Can you work these out from the model? Positions are in its coordinate system, mm. Face numbers are marked on the shaded views. Give positions to 0.01 mm unless a question says otherwise; leave off trailing zeros. Loops run counter-clockwise (first coordinate to the right, second up) from the corner with the lowest first, then second, coordinate; pieces in that order, holes last. Notation, with made-up numbers: (59.5, 48.5) -> (71.5, 48.5) arc R20 cw to (71.5, 76.5) -> close; hole circle Ø5 at (-5, 63.5). An arc over 180 degrees is marked (long way). Return JSON: item names as keys, results as strings. Group by question number.
Q1. Suppose I cut it at B-B, the plane y = 35. Please give me the cut outline in (x, z), and give its area (3 significant figures).
Q2. Thinking about a two-plate mould opening in X: for the marked faces 1 and 2, which applies, pulls with the +X half, pulls with the -X half, needs draft (parallel to the pull), parting line crosses it, or undercut?
Q3. Will these pins go through, and if not, where does the flat tip stop? pin 1 (1 mm diameter, centred on x = 53.5, z = 5, fed in from -Y); pin 2 (14.5 mm diameter, centred on x = 42, y = -24, fed in from +Z); pin 3 (6 mm diameter, centred on x = -60.5, y = -53, fed in from -Z).
Q4. Suppose I cut it at A-A, the plane z = -4.5. Please give me the cut outline in (x, y), and give its area (3 significant figures).
Q5. Suppose I cut it at D-D, the plane y = 11. Please give me the cut outline in (x, z), and give its area (3 significant figures).
Q6. Suppose I cut it at C-C, the plane x = 66.5. Please give me the cut outline in (y, z), and give its area (3 significant figures).
Q7. I need wall thicknesses on line 1 along Y through (x, z) = (8, -6.5); line 2 along Z through (x, y) = (57, 61). Which ranges of each line are inside material? Lowest first, please. Write a range as [from, to].
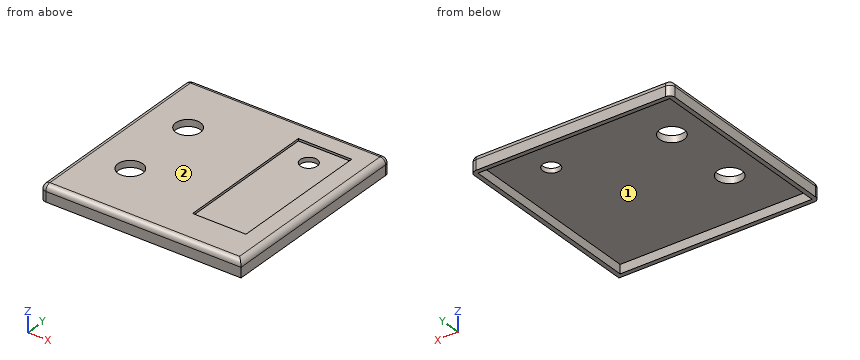
```python
from build123d import *

# Parameters (mm, degrees)
F0_W     = 180
F0_H     = 180
F0_R     = 11.1125
F0_W_2   = 47.792598
F0_H_2   = 127.960831
F1_DEPTH = 6
F0_R_2   = 7.62
F2_DEPTH = 4
F3_W     = 180
F3_H     = 180
F3_W_2   = 172
F3_H_2   = 172
F4_DEPTH = 8
F5_R     = 5


with BuildPart() as f1:
    # F0 (on Top) → F1 (new body)
    with BuildSketch(Plane.XY):
        Rectangle(F0_W, F0_H)
        with Locations((-50.008792, -35)):
            Circle(F0_R, mode=Mode.SUBTRACT)
        with Locations((-50.008792, 35)):
            Circle(F0_R, mode=Mode.SUBTRACT)
        with Locations((46.732679, 6.070435)):
            Rectangle(F0_W_2, F0_H_2, mode=Mode.SUBTRACT)
    extrude(amount=F1_DEPTH)

    # F0 (on Top) → F2 (join)
    with BuildSketch(Plane.XY):
        with Locations((46.732679, 6.070435)):
            Rectangle(F0_W_2, F0_H_2)
        with Locations((46.732679, 50.394215)):
            Circle(F0_R_2, mode=Mode.SUBTRACT)
    extrude(amount=F2_DEPTH)

    # F3 (on Top) → F4 (join)
    with BuildSketch(Plane.XY):
        Rectangle(F3_W, F3_H)
        Rectangle(F3_W_2, F3_H_2, mode=Mode.SUBTRACT)
    extrude(amount=-F4_DEPTH)

    # F5
    f5_edges = [f1.edges().sort_by_distance(p)[0] for p in [
        (-90, 0, 6),
        (0, -90, 6),
        (90, 0, 6),
        (90, 90, -1),
        (0, 90, 6),
        (-90, 90, -1),
        (-90, -90, -1),
    ]]
    fillet(f5_edges, radius=F5_R)


solid = f1.part
```
Ans:
{
 "1": {"outline": "(-90, -8) -> (-86, -8) -> (-86, 0) -> (-61.12, 0) -> (-61.12, 6) -> (-85, 6) arc R5 ccw to (-90, 1) -> close; (-38.9, 0) -> (86, 0) -> (86, -8) -> (90, -8) -> (90, 1) arc R5 ccw to (85, 6) -> (70.63, 6) -> (70.63, 4) -> (22.84, 4) -> (22.84, 6) -> (-38.9, 6) -> close", "area": "904 mm^2"},
 "2": {"face 1": "undercut", "face 2": "needs draft"},
 "3": {"pin 1": "stops at y = -88.57", "pin 2": "stops at z = 4", "pin 3": "stops at z = 0"},
 "4": {"outline": "(-90, -85) arc R5 ccw to (-85, -90) -> (90, -90) -> (90, 85) arc R5 ccw to (85, 90) -> (-85, 90) arc R5 ccw to (-90, 85) -> close; hole (-86, -86) -> (86, -86) -> (86, 86) -> (-86, 86) -> close", "area": "2,800 mm^2"},
 "5": {"outline": "(-90, -8) -> (-86, -8) -> (-86, 0) -> (86, 0) -> (86, -8) -> (90, -8) -> (90, 1) arc R5 ccw to (85, 6) -> (70.63, 6) -> (70.63, 4) -> (22.84, 4) -> (22.84, 6) -> (-85, 6) arc R5 ccw to (-90, 1) -> close", "area": "1,040 mm^2"},
 "6": {"outline": "(-90, -8) -> (-86, -8) -> (-86, 0) -> (86, 0) -> (86, -8) -> (90, -8) -> (90, 1) arc R5 ccw to (85, 6) -> (70.05, 6) -> (70.05, 4) -> (-57.91, 4) -> (-57.91, 6) -> (-85, 6) arc R5 ccw to (-90, 1) -> close", "area": "877 mm^2"},
 "7": {"line 1": "y = [-90, -86], [86, 90]", "line 2": "z = [0, 4]"}
}
